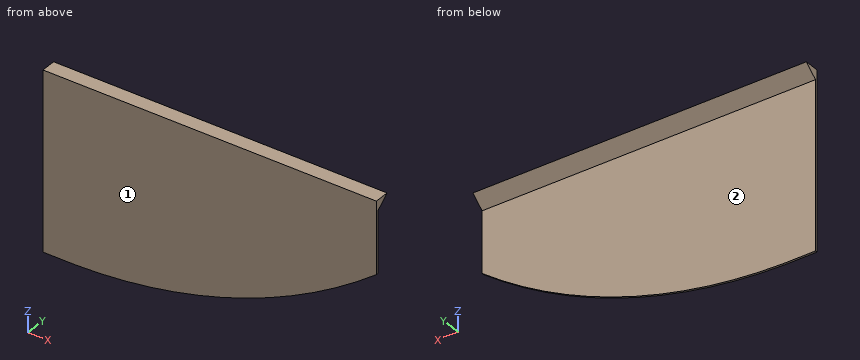
```python
from build123d import *

# Parameters (mm, degrees)
F1_DEPTH = 2.54
F2_W     = 398.78
F2_H     = 12.7
F3_DEPTH = 15.24
F5_DEPTH = 406.4


with BuildPart() as f1:
    # F0 (on Front) → F1 (new body)
    with BuildSketch(Plane.XZ):
        with BuildLine():
            Line((210.516836579, -71.3362430625), (-188.263163421, -71.3362430625))
            Line((-188.263163421, -71.3362430625), (-188.263163421, -139.4082430625))
            Line((-188.263163421, -139.4082430625), (-188.263163421, -284.1882430625))
            Line((-188.263163421, -284.1882430625), (-172.261163421, -284.1882430625))
            Line((-172.261163421, -284.1882430625), (-149.3573673049, -284.1882430625))
            ThreePointArc((-149.3573673049, -284.1882430625), (40.8389414751, -249.7592973406), (210.516836579, -157.1882430625))
            Line((210.516836579, -157.1882430625), (210.516836579, -71.3362430625))
        make_face()
    extrude(amount=F1_DEPTH)

    # F2 (on face) → F3 (join)
    with BuildSketch(Plane(origin=(0, 0, 0), x_dir=(-1, 0, 0), z_dir=(0, 1, 0))):
        with Locations((-11.126836579, -77.6862430625)):
            Rectangle(F2_W, F2_H)
    extrude(amount=F3_DEPTH)

    # F4 (on face) → F5 (cut)
    with BuildSketch(Plane.YZ.offset(210.516836579)):
        Polygon((15.24, -71.3362430625), (0, -84.0362430625), (15.24, -84.0362430625), align=None)
    extrude(amount=-F5_DEPTH, mode=Mode.SUBTRACT)


solid = f1.part
```
Part model, mm, in its own coordinate system. Face numbers are marked on the shaded views. A direction names the side the tool comes from. Coordinates: 2 decimals unless noted, no trailing zeros. Write each loop counter-clockwise with the first axis right and the second up, starting at its lowest first coordinate (ties: lowest second). Pieces come first, ordered by that corner, then holes.
Item 1: Slice it at C-C (y = 4). Write the cut outline in (x, z), and give its area (3 significant figures).
Item 2: Slice it at D-D (x = -158). Write the cut outline in (y, z), and give its area (3 significant figures).
Item 3: Which spindle directions (+Z, -Z, +X, -X, +Y, -Y) get a long thin tool onto all of the face, cutting with end or side? Do the marked faces 1 and 2. Say none if no direction does.
Item 4: Probe line 1 (Y direction, x = -26, z = -112.5); line 2 (Z direction, x = -156.5, y = 3.5); line 3 (Z direction, x = 33, y = 9). List the from-to ranges inside material, lowest first.
Item 5: Pin check, flat tips, straight feed: pin 1 (6 mm diameter, centred on x = 151.5, y = 2, fed in from -Z); pin 2 (5 mm diameter, centred on y = -0.5, z = -196.5, fed in from +X); pin 3 (6 mm diameter, centred on x = 38.5, z = -154, fed in from +Y). Stop position of each tip, or through.
Item 6: Slice it at A-A (x = 79.5). Write the cut outline in (y, z).
Item 7: Slice it at B-B (z = -242). Write the cut outline in (x, y), and give its area (3 significant figures).
Results found:
1. outline: (-188.26, -80.7) - (210.52, -80.7) - (210.52, -71.34) - (-188.26, -71.34) - close
1. area: 3,740 mm2
2. outline: (-2.54, -284.19) - (0, -284.19) - (0, -84.04) - (15.24, -71.34) - (-2.54, -71.34) - close
2. area: 637 mm2
3. face 1: +Z, -Z, +X, -X, -Y
3. face 2: -Z, +X, -X, +Y
4. line 1: y = -2.54 to 0
4. line 2: z = -81.12 to -71.34
4. line 3: z = -76.54 to -71.34
5. pin 1: stops at z = -198.95
5. pin 2: stops at x = 157.43
5. pin 3: stops at y = 0
6. outline: (-2.54, -234.61) - (0, -234.61) - (0, -84.04) - (15.24, -71.34) - (-2.54, -71.34) - close
7. outline: (-188.26, -2.54) - (61.61, -2.54) - (61.61, 0) - (-188.26, 0) - close
7. area: 635 mm2
